Geometry: final body of the model. Coordinates: model frame, mm. A direction names the side the tool comes from. Give positions to 0.01 mm unless a question says otherwise; leave off trailing zeros. Loops run counter-clockwise (first coordinate to the right, second up) from the corner with the lowest first, then second, coordinate; pieces in that order, holes last. Notation, with made-up numbers: M 57.5,42 L 90.5,42 A24 cw 90.5,74 Z; hole C 9,7 d9. An arc over 180 degrees is marked long. Put each result on its own line as item: value.
```python
from build123d import *

# Parameters (mm, degrees)
SKETCH1_R                = 1
BOSS_EXTRUDE1_DEPTH      = 10
BOSS_EXTRUDE2_DEPTH      = 1
BOSS_EXTRUDE2_DEPTH_BACK = 1
FILLET1_R                = 1
SKETCH3_R                = 0.6
CUT_EXTRUDE1_DEPTH       = 5


with BuildPart() as part:
    # Sketch1 → Boss-Extrude1 (new body)
    with BuildSketch(Plane(origin=(0, 0, 0), x_dir=(0, 0, -1), z_dir=(1, 0, 0))):
        Circle(SKETCH1_R)
    extrude(amount=BOSS_EXTRUDE1_DEPTH)

    # Sketch2 → Boss-Extrude2 (add, two sides: drawn at the far end of the back side and taken through both)
    with BuildSketch(Plane(origin=(0, 0, 0), x_dir=(1, 0, 0), z_dir=(0, 1, 0)).offset(-BOSS_EXTRUDE2_DEPTH_BACK)):
        Polygon((1, 1.875), (1, -1.875), (-3, -1.875), (-3, -0.875), (0, -0.875), (0, 0.875), (-3, 0.875), (-3, 1.875), align=None)
    extrude(amount=BOSS_EXTRUDE2_DEPTH + BOSS_EXTRUDE2_DEPTH_BACK)

    # Fillet1
    fillet1_edges = [part.edges().sort_by_distance(p)[0] for p in [
        (-3, 1, -1.375),
        (-3, -1, -1.375),
        (-3, -1, 1.375),
        (-3, 1, 1.375),
        (1, 0, -1.875),
        (1, 0, 1.875),
    ]]
    fillet(fillet1_edges, radius=FILLET1_R - 0.0001)  # a hair under: the kernel refuses the full size

    # Sketch3 → Cut-Extrude1 (cut)
    with BuildSketch(Plane(origin=(0, 0, -1.875), x_dir=(-1, 0, 0), z_dir=(0, 0, -1))):
        with Locations((1.7, 0)):
            Circle(SKETCH3_R)
    extrude(amount=-CUT_EXTRUDE1_DEPTH, mode=Mode.SUBTRACT)


solid = part.part
```
Item 1: Mould query, pull axis Z, two halves, no side actions, for faces 1 (the flat face through (-1.1, -0.5, -0.875)), 2 (the cylindrical face through (-1.1, 0, -1.4)), 3 (the cylindrical face through (0.7, 0.75, 1.59)). Classes: pulls with the +Z half, pulls with the -Z half, needs draft (parallel to the pull), parting line crosses it, or undercut.
Output values:
face 1: undercut
face 2: needs draft
face 3: pulls with the +Z half
Item 2: Line query: probe 1 along Y at (x, z) = (-1.7, -1.6); probe 2 along Z at (x, y) = (-1, -0.6) (3 decimals); probe 3 along X at (y, z) = (-0.6, 0.2). Output: solid intervals per line, ascending. Write a range as [from, to].
Output values:
probe 1: [-1, -0.6], [0.6, 1]
probe 2: [-1.875, -0.875], [0.875, 1.875]
probe 3: [0, 10]
Item 3: Section C-C on y = -0.8. Output: boundary loops of the cut face in (x, z) (3 decimals), then the cut area to 3 significant figures.
Output values:
outline: M -2.6,-1.875 L 0,-1.875 A1 ccw 1,-0.875 L 1,-0.6 L 10,-0.6 L 10,0.6 L 1,0.6 L 1,0.875 A1 ccw 0,1.875 L -2.6,1.875 L -2.6,0.875 L 0,0.875 L 0,-0.875 L -2.6,-0.875 Z
area: 19.3 mm²
Item 4: Section A-A on x = -1.7. Output: boundary loops of the cut face in (y, z) (3 decimals), then the cut area to 3 significant figures.
Output values:
outline: M -1,-1.875 L -0.6,-1.875 L -0.6,-0.875 L -1,-0.875 Z; M -1,0.875 L -0.6,0.875 L -0.6,1.875 L -1,1.875 Z; M 0.6,-1.875 L 1,-1.875 L 1,-0.875 L 0.6,-0.875 Z; M 0.6,0.875 L 1,0.875 L 1,1.875 L 0.6,1.875 Z
area: 1.60 mm²
Item 5: Section B-B on z = 0.75. Output: boundary loops of the cut face in (x, y).
Output values:
outline: M 0,-1 L 1,-1 L 1,-0.66 L 10,-0.66 L 10,0.66 L 1,0.66 L 1,1 L 0,1 Z
Item 6: Section D-D on y = -0.2. Count the separate pieces of the cut face and the enclosed holes in it, then the cut area to 3 significant figures.
Output values:
separate pieces: 3
enclosed holes: 0
area: 24.7 mm²
Item 7: Set-up query: faces 4 (the cylindrical face through (0.7, -0.74, 1.59)), 5 (the cylindrical face through (0.715, 0.746, -1.574)), 6 (the cylindrical face through (0.715, -0.738, -1.574)), 7 (the flat face through (-0.9, 0, 0.875)). Return all of +Z, -Z, +X, -X, +Y, -Y with unobstructed straight access to the full face (end or side cutting, diameter ignored); none if empty.
Output values:
face 4: +Z, +X, -Y
face 5: -Z, +X, +Y
face 6: -Z, +X, -Y
face 7: -X, +Y, -Y
Item 8: Pin query (flat end, axial travel): pin 1 Ø1 at (x, z) = (5, -1) entering from -Y; pin 2 Ø0.5 at (y, z) = (0.5, -0.5) entering from -X. Return the tip coordinate at first contact, or that it passes through.
Output values:
pin 1: y = -0.87
pin 2: x = 0
